Source: CAD feature listing. Evaluate the final solid. Frame: model axes, mm. A direction names the side the tool comes from. Give positions to 0.01 mm unless a question says otherwise; leave off trailing zeros. Order: outer loops, then holes, each group sorted by start corner. A loop starts at its lowest first (then second) coordinate and runs counter-clockwise, first axis right, second up. Notation, with made-up numbers: M 11,-17 L 65,-17 A25 ccw 65,10 Z; hole C 19,79 d10. An arc over 180 degrees is marked long. Answer in a Markdown table with one row per item. Add a question column.
(1) Mould query, pull axis X, two halves, no side actions, for faces 1 (the face through (74, 10, -55)), 2 (the face through (155, 16, -5)), 3 (the face through (152, 35, -2)), 4 (the face through (0, 59, -59)). Classes: pulls with the +X half, pulls with the -X half, needs draft (parallel to the pull), parting line crosses it, or undercut.
(2) Section query C-C, the plane x = 20. Return loops of the section in (y, z).
(3) Section query D-D, the plane z = -100. Return loops of the section in (x, y).
(4) Section query A-A, the plane y = 49.5. Return loops of the section in (x, z), plus the area to 3 significant figures.
(5) Material intervals for line 1 along X through (y, z) = (56.5, -70); line 2 along X through (y, z) = (60, -100); line 3 along Z through (x, y) = (20, 4), sorted ascending.
(6) Section query B-B, the plane z = -57. Return loops of the section in (x, y), plus the area to 3 significant figures.
(7) Set-up query: faces 5 (the face through (152, 31.215, -5)), 6 (the face through (152, 25, -2)), 7 (the face through (113.682, 64.23, -93.855)). Return all of +Z, -Z, +X, -X, +Y, -Y with unobstructed straight access to the full face (end or side cutting, diameter ignored); none if empty.
(8) Pin query (flat end, axial travel): P1, Ø10, axis at x = 43, z = -44.5, coming from the +Y side; P2, Ø5.5, axis at x = 153, y = 35.5, coming from the -Z side; P3, Ø1, axis at y = 22, z = -108, coming from the +X side; P4, Ø4, axis at y = 23.5, z = -65.5, coming from the -X side. Return the tip coordinate at first contact, or that it passes through.
from build123d import *

# Parameters (mm, degrees)
SKETCH1_W                = 150
SKETCH1_H                = 120
BASEBOX_DEPTH            = 120
SKETCH2_W                = 130
SKETCH2_H                = 110
INTERIORCUT_DEPTH        = 110
POSITIONCALIBRATOR_DEPTH = 110
SKETCH6_W                = 6.959896851
SKETCH6_H                = 7.60749883
LASERRECEIVER_DEPTH      = 5
THREADEDROD_DEPTH        = 225.77766793
THREADEDROD_DEPTH_BACK   = 225.77766793
SKETCH3_R                = 5


with BuildPart() as part:
    # Sketch1 → BaseBox (new body)
    with BuildSketch(Plane(origin=(0, 0, 0), x_dir=(1, 0, 0), z_dir=(0, 1, 0))):
        with Locations((75, 60)):
            Rectangle(SKETCH1_W, SKETCH1_H)
    extrude(amount=BASEBOX_DEPTH)

    # Sketch2 → InteriorCut (cut)
    with BuildSketch(Plane(origin=(0, 120, 0), x_dir=(1, 0, 0), z_dir=(0, 1, 0))):
        with Locations((75, 55)):
            Rectangle(SKETCH2_W, SKETCH2_H)
    extrude(amount=-INTERIORCUT_DEPTH, mode=Mode.SUBTRACT)

    # Sketch5 → PositionCalibrator (add)
    with BuildSketch(Plane(origin=(0, 10, 0), x_dir=(1, 0, 0), z_dir=(0, 1, 0))):
        with BuildLine():
            Line((63.383989491, 97.819381253), (10, 90))
            Line((10, 90), (10, 110))
            Line((10, 110), (140, 110))
            Line((140, 110), (140, 90))
            Line((140, 90), (86.616010509, 97.819381253))
            ThreePointArc((86.616010509, 97.819381253), (75, 109.435391763), (63.383989491, 97.819381253))
        make_face()
    extrude(amount=POSITIONCALIBRATOR_DEPTH)

    # Sketch6 → LaserReceiver (add)
    with BuildSketch(Plane(origin=(150, 0, 0), x_dir=(0, 0, -1), z_dir=(1, 0, 0))):
        with Locations((5.479948425, 35.018747075)):
            Rectangle(SKETCH6_W, SKETCH6_H)
        with Locations((5.479948425, 15.803749415)):
            Rectangle(SKETCH6_W, SKETCH6_H)
        with Locations((5.479948425, 25.411248245)):
            Rectangle(SKETCH6_W, SKETCH6_H)
    extrude(amount=LASERRECEIVER_DEPTH)

    # Sketch3 → ThreadedRod (cut, two sides: drawn at the far end of the back side and taken through both)
    with BuildSketch(Plane(origin=(0, 10, 0), x_dir=(1, 0, 0), z_dir=(0, 1, 0)).offset(-THREADEDROD_DEPTH_BACK)):
        with Locations(Location((20, 10, 0), (0, 0, 270))):
            Circle(SKETCH3_R)
        with Locations(Location((130, 100, 0), (0, 0, 270))):
            Circle(SKETCH3_R)
    extrude(amount=THREADEDROD_DEPTH + THREADEDROD_DEPTH_BACK, mode=Mode.SUBTRACT)


solid = part.part
Values follow:
| question | item | result |
|---|---|---|
| 1 | face 1 | undercut |
| 1 | face 2 | pulls with the +X half |
| 1 | face 3 | needs draft |
| 1 | face 4 | pulls with the -X half |
| 2 | outline | M 0,-120 L 120,-120 L 120,-91.46 L 10,-91.46 L 10,-15 L 0,-15 Z; M 0,-5 L 10,-5 L 10,0 L 0,0 Z |
| 3 | outline | M 0,0 L 125,0 L 125,120 L 86.41,120 L 86.41,10 L 63.59,10 L 63.59,120 L 0,120 Z; M 135,0 L 150,0 L 150,120 L 135,120 Z |
| 4 | outline | M 0,-120 L 150,-120 L 150,0 L 140,0 L 140,-90 L 86.62,-97.82 A11.62 cw 63.38,-97.82 L 10,-90 L 10,0 L 0,0 Z; hole C 130,-100 d10 |
| 4 | area | 5,410 mm² |
| 5 | line 1 | x = 0 to 10, 140 to 150 |
| 5 | line 2 | x = 0 to 63.59, 86.41 to 125, 135 to 150 |
| 5 | line 3 | z = -120 to -15, -5 to 0 |
| 6 | outline | M 0,0 L 150,0 L 150,120 L 140,120 L 140,10 L 10,10 L 10,120 L 0,120 Z |
| 6 | area | 3,700 mm² |
| 7 | face 5 | +Z, -Z, +X |
| 7 | face 6 | +Z, +X, +Y, -Y |
| 7 | face 7 | +Z, +Y |
| 8 | P1 | stops at y = 10 |
| 8 | P2 | stops at z = -8.96 |
| 8 | P3 | stops at x = 150 |
| 8 | P4 | stops at x = 0 |
